```python
from build123d import *

# Parameters (mm, degrees)
SKETCH_1_R       = 8
EXTRUDE_1_DEPTH  = 24
SKETCH_2_R       = 17.5
SKETCH_2_R_2     = 8
EXTRUDE_2_DEPTH  = 18
EXTRUDE_3_DEPTH  = 18
EXTRUDE_4_DEPTH  = 18
EXTRUDE_5_DEPTH  = 18
EXTRUDE_6_DEPTH  = 18
EXTRUDE_7_DEPTH  = 18
EXTRUDE_8_DEPTH  = 18
EXTRUDE_9_DEPTH  = 18
EXTRUDE_10_DEPTH = 18
EXTRUDE_11_DEPTH = 18
EXTRUDE_12_DEPTH = 18
EXTRUDE_13_DEPTH = 18
EXTRUDE_14_DEPTH = 18
EXTRUDE_15_DEPTH = 18
EXTRUDE_16_DEPTH = 18
EXTRUDE_17_DEPTH = 18
EXTRUDE_18_DEPTH = 18
EXTRUDE_19_DEPTH = 18
EXTRUDE_20_DEPTH = 18
EXTRUDE_21_DEPTH = 18
EXTRUDE_22_DEPTH = 18


with BuildPart() as part:
    # 草图1 → 凸台-拉伸1 (new body)
    with BuildSketch(Plane.XY):
        Circle(SKETCH_1_R)
        with BuildLine():
            Line((4.520101179, 2.361924075), (-4.833937562, 1.62574526))
            ThreePointArc((-4.833937562, 1.62574526), (0.400141388, -5.084278402), (4.520101179, 2.361924075))
        make_face(mode=Mode.SUBTRACT)
    extrude(amount=EXTRUDE_1_DEPTH)

    # 草图2 → 凸台-拉伸2 (add)
    with BuildSketch(Plane.XY):
        Circle(SKETCH_2_R)
        Circle(SKETCH_2_R_2, mode=Mode.SUBTRACT)
    extrude(amount=EXTRUDE_2_DEPTH)

    # 草图3 → 凸台-拉伸3 (add)
    with BuildSketch(Plane.XY):
        with BuildLine():
            Line((17.423652167, 1.632894724), (21.989026862, 0.69476445))
            ThreePointArc((21.989026862, 0.69476445), (22, 0), (21.989026862, -0.69476445))
            Line((21.989026862, -0.69476445), (17.423652167, -1.632894724))
            ThreePointArc((17.423652167, -1.632894724), (17.5, 0), (17.423652167, 1.632894724))
        make_face()
    extrude(amount=EXTRUDE_3_DEPTH)

    # 草图4 → 凸台-拉伸4 (add)
    with BuildSketch(Plane.XY):
        with BuildLine():
            Line((16.066285711, 6.937179791), (20.698113262, 7.455743248))
            ThreePointArc((20.698113262, 7.455743248), (20.923243358, 6.798373876), (21.127501307, 6.134222733))
            Line((21.127501307, 6.134222733), (17.07547015, 3.831229456))
            ThreePointArc((17.07547015, 3.831229456), (16.643489035, 5.407797402), (16.066285711, 6.937179791))
        make_face()
    extrude(amount=EXTRUDE_4_DEPTH)

    # 草图5 → 凸台-拉伸5 (add)
    with BuildSketch(Plane.XY):
        with BuildLine():
            Line((13.13623927, 11.562405366), (17.381124124, 13.486901949))
            ThreePointArc((17.381124124, 13.486901949), (17.798373876, 12.93127555), (18.197868719, 12.362749455))
            Line((18.197868719, 12.362749455), (15.055822144, 8.920326203))
            ThreePointArc((15.055822144, 8.920326203), (14.157797402, 10.286241915), (13.13623927, 11.562405366))
        make_face()
    extrude(amount=EXTRUDE_5_DEPTH)

    # 草图6 → 凸台-拉伸6 (add)
    with BuildSketch(Plane.XY):
        with BuildLine():
            Line((8.920326203, 15.055822144), (12.212561116, 18.348057057))
            ThreePointArc((12.212561116, 18.348057057), (12.870731845, 17.892515435), (13.511927681, 17.413375811))
            Line((13.511927681, 17.413375811), (11.562405366, 13.13623927))
            ThreePointArc((11.562405366, 13.13623927), (10.286241915, 14.157797402), (8.920326203, 15.055822144))
        make_face()
    extrude(amount=EXTRUDE_6_DEPTH)

    # 草图7 → 凸台-拉伸7 (add)
    with BuildSketch(Plane.XY):
        with BuildLine():
            Line((3.831229456, 17.07547015), (6.134222733, 21.127501307))
            ThreePointArc((6.134222733, 21.127501307), (6.798373876, 20.923243358), (7.455743248, 20.698113262))
            Line((7.455743248, 20.698113262), (6.937179791, 16.066285711))
            ThreePointArc((6.937179791, 16.066285711), (5.407797402, 16.643489035), (3.831229456, 17.07547015))
        make_face()
    extrude(amount=EXTRUDE_7_DEPTH)

    # 草图8 → 凸台-拉伸8 (add)
    with BuildSketch(Plane.XY):
        with BuildLine():
            Line((-1.632894724, 17.423652167), (-0.69476445, 21.989026862))
            ThreePointArc((-0.69476445, 21.989026862), (0, 22), (0.69476445, 21.989026862))
            Line((0.69476445, 21.989026862), (1.632894724, 17.423652167))
            ThreePointArc((1.632894724, 17.423652167), (0, 17.5), (-1.632894724, 17.423652167))
        make_face()
    extrude(amount=EXTRUDE_8_DEPTH)

    # 草图9 → 凸台-拉伸9 (add)
    with BuildSketch(Plane.XY):
        with BuildLine():
            Line((-6.937179791, 16.066285711), (-7.455743248, 20.698113262))
            ThreePointArc((-7.455743248, 20.698113262), (-6.798373876, 20.923243358), (-6.134222733, 21.127501307))
            Line((-6.134222733, 21.127501307), (-3.831229456, 17.07547015))
            ThreePointArc((-3.831229456, 17.07547015), (-5.407797402, 16.643489035), (-6.937179791, 16.066285711))
        make_face()
    extrude(amount=EXTRUDE_9_DEPTH)

    # 草图10 → 凸台-拉伸10 (add)
    with BuildSketch(Plane.XY):
        with BuildLine():
            Line((-11.562405366, 13.13623927), (-13.486901949, 17.381124124))
            ThreePointArc((-13.486901949, 17.381124124), (-12.93127555, 17.798373876), (-12.362749455, 18.197868719))
            Line((-12.362749455, 18.197868719), (-8.920326203, 15.055822144))
            ThreePointArc((-8.920326203, 15.055822144), (-10.286241915, 14.157797402), (-11.562405366, 13.13623927))
        make_face()
    extrude(amount=EXTRUDE_10_DEPTH)

    # 草图11 → 凸台-拉伸11 (add)
    with BuildSketch(Plane.XY):
        with BuildLine():
            Line((-15.055822144, 8.920326203), (-18.348057057, 12.212561116))
            ThreePointArc((-18.348057057, 12.212561116), (-17.892515435, 12.870731845), (-17.413375811, 13.511927681))
            Line((-17.413375811, 13.511927681), (-13.13623927, 11.562405366))
            ThreePointArc((-13.13623927, 11.562405366), (-14.157797402, 10.286241915), (-15.055822144, 8.920326203))
        make_face()
    extrude(amount=EXTRUDE_11_DEPTH)

    # 草图12 → 凸台-拉伸12 (add)
    with BuildSketch(Plane.XY):
        with BuildLine():
            Line((-17.07547015, 3.831229456), (-21.127501307, 6.134222733))
            ThreePointArc((-21.127501307, 6.134222733), (-20.923243358, 6.798373876), (-20.698113262, 7.455743248))
            Line((-20.698113262, 7.455743248), (-16.066285711, 6.937179791))
            ThreePointArc((-16.066285711, 6.937179791), (-16.643489035, 5.407797402), (-17.07547015, 3.831229456))
        make_face()
    extrude(amount=EXTRUDE_12_DEPTH)

    # 草图13 → 凸台-拉伸13 (add)
    with BuildSketch(Plane.XY):
        with BuildLine():
            Line((-17.423652167, -1.632894724), (-21.989026862, -0.69476445))
            ThreePointArc((-21.989026862, -0.69476445), (-22, 0), (-21.989026862, 0.69476445))
            Line((-21.989026862, 0.69476445), (-17.423652167, 1.632894724))
            ThreePointArc((-17.423652167, 1.632894724), (-17.5, 0), (-17.423652167, -1.632894724))
        make_face()
    extrude(amount=EXTRUDE_13_DEPTH)

    # 草图14 → 凸台-拉伸14 (add)
    with BuildSketch(Plane.XY):
        with BuildLine():
            Line((-16.066285711, -6.937179791), (-20.698113262, -7.455743248))
            ThreePointArc((-20.698113262, -7.455743248), (-20.923243358, -6.798373876), (-21.127501307, -6.134222733))
            Line((-21.127501307, -6.134222733), (-17.07547015, -3.831229456))
            ThreePointArc((-17.07547015, -3.831229456), (-16.643489035, -5.407797402), (-16.066285711, -6.937179791))
        make_face()
    extrude(amount=EXTRUDE_14_DEPTH)

    # 草图15 → 凸台-拉伸15 (add)
    with BuildSketch(Plane.XY):
        with BuildLine():
            Line((-13.13623927, -11.562405366), (-17.381124124, -13.486901949))
            ThreePointArc((-17.381124124, -13.486901949), (-17.798373876, -12.93127555), (-18.197868719, -12.362749455))
            Line((-18.197868719, -12.362749455), (-15.055822144, -8.920326203))
            ThreePointArc((-15.055822144, -8.920326203), (-14.157797402, -10.286241915), (-13.13623927, -11.562405366))
        make_face()
    extrude(amount=EXTRUDE_15_DEPTH)

    # 草图16 → 凸台-拉伸16 (add)
    with BuildSketch(Plane.XY):
        with BuildLine():
            Line((-8.920326203, -15.055822144), (-12.212561116, -18.348057057))
            ThreePointArc((-12.212561116, -18.348057057), (-12.870731845, -17.892515435), (-13.511927681, -17.413375811))
            Line((-13.511927681, -17.413375811), (-11.562405366, -13.13623927))
            ThreePointArc((-11.562405366, -13.13623927), (-10.286241915, -14.157797402), (-8.920326203, -15.055822144))
        make_face()
    extrude(amount=EXTRUDE_16_DEPTH)

    # 草图17 → 凸台-拉伸17 (add)
    with BuildSketch(Plane.XY):
        with BuildLine():
            Line((-3.831229456, -17.07547015), (-6.134222733, -21.127501307))
            ThreePointArc((-6.134222733, -21.127501307), (-6.798373876, -20.923243358), (-7.455743248, -20.698113262))
            Line((-7.455743248, -20.698113262), (-6.937179791, -16.066285711))
            ThreePointArc((-6.937179791, -16.066285711), (-5.407797402, -16.643489035), (-3.831229456, -17.07547015))
        make_face()
    extrude(amount=EXTRUDE_17_DEPTH)

    # 草图18 → 凸台-拉伸18 (add)
    with BuildSketch(Plane.XY):
        with BuildLine():
            Line((1.632894724, -17.423652167), (0.69476445, -21.989026862))
            ThreePointArc((0.69476445, -21.989026862), (0, -22), (-0.69476445, -21.989026862))
            Line((-0.69476445, -21.989026862), (-1.632894724, -17.423652167))
            ThreePointArc((-1.632894724, -17.423652167), (0, -17.5), (1.632894724, -17.423652167))
        make_face()
    extrude(amount=EXTRUDE_18_DEPTH)

    # 草图19 → 凸台-拉伸19 (add)
    with BuildSketch(Plane.XY):
        with BuildLine():
            Line((6.937179791, -16.066285711), (7.455743248, -20.698113262))
            ThreePointArc((7.455743248, -20.698113262), (6.798373876, -20.923243358), (6.134222733, -21.127501307))
            Line((6.134222733, -21.127501307), (3.831229456, -17.07547015))
            ThreePointArc((3.831229456, -17.07547015), (5.407797402, -16.643489035), (6.937179791, -16.066285711))
        make_face()
    extrude(amount=EXTRUDE_19_DEPTH)

    # 草图20 → 凸台-拉伸20 (add)
    with BuildSketch(Plane.XY):
        with BuildLine():
            Line((11.562405366, -13.13623927), (13.486901949, -17.381124124))
            ThreePointArc((13.486901949, -17.381124124), (12.93127555, -17.798373876), (12.362749455, -18.197868719))
            Line((12.362749455, -18.197868719), (8.920326203, -15.055822144))
            ThreePointArc((8.920326203, -15.055822144), (10.286241915, -14.157797402), (11.562405366, -13.13623927))
        make_face()
    extrude(amount=EXTRUDE_20_DEPTH)

    # 草图21 → 凸台-拉伸21 (add)
    with BuildSketch(Plane.XY):
        with BuildLine():
            Line((15.055822144, -8.920326203), (18.348057057, -12.212561116))
            ThreePointArc((18.348057057, -12.212561116), (17.892515435, -12.870731845), (17.413375811, -13.511927681))
            Line((17.413375811, -13.511927681), (13.13623927, -11.562405366))
            ThreePointArc((13.13623927, -11.562405366), (14.157797402, -10.286241915), (15.055822144, -8.920326203))
        make_face()
    extrude(amount=EXTRUDE_21_DEPTH)

    # 草图22 → 凸台-拉伸22 (add)
    with BuildSketch(Plane.XY):
        with BuildLine():
            Line((17.07547015, -3.831229456), (21.127501307, -6.134222733))
            ThreePointArc((21.127501307, -6.134222733), (20.923243358, -6.798373876), (20.698113262, -7.455743248))
            Line((20.698113262, -7.455743248), (16.066285711, -6.937179791))
            ThreePointArc((16.066285711, -6.937179791), (16.643489035, -5.407797402), (17.07547015, -3.831229456))
        make_face()
    extrude(amount=EXTRUDE_22_DEPTH)


solid = part.part
```
Input: part model. Units: mm. Frame: model coordinates. A direction names the side the tool comes from. Round coordinates to 2 decimals unless told otherwise and drop trailing zeros. Write each loop counter-clockwise with the first axis right and the second up, starting at its lowest first coordinate (ties: lowest second). Pieces come first, ordered by that corner, then holes. Notation, with made-up numbers: (18, 70.25) -> (23, 70.25) arc R5 ccw to (23, 77.25) -> close; hole circle Ø5 at (38, -3). An arc over 180 degrees is marked (long way). Answer as CSV lines item,"result".
1. Reachability of faces 1 (the flat face through (4.967, 19.073, 8.874)), 2 (the cylindrical face through (-7.959, -15.586, 8.874)), 3 (the flat face through (5, -19.13, 8.87)), 4 (the flat face through (-9, 0, 18)) from +Z, -Z, +X, -X, +Y, -Y: full face, straight path, thin tool, end or side. Return the list, or none.
Geometry says:
face 1,"+Z, -Z, +Y"
face 2,"+Z, -Z"
face 3,"+Z, -Z, -Y"
face 4,"+Z"
2. Section C-C (y = -19). Return the cut outline in (x, z).
Geometry says:
outline,"(-7.27, 0) -> (-4.93, 0) -> (-4.93, 18) -> (-7.27, 18) -> close; (-1.31, 0) -> (1.31, 0) -> (1.31, 18) -> (-1.31, 18) -> close; (4.93, 0) -> (7.27, 0) -> (7.27, 18) -> (4.93, 18) -> close"
3. Ray query, L1, parallel to X at y = 0, z = 5.25; L2, parallel to X at y = -12.5, z = 8; L3, parallel to Z at x = -15, y = 8.5. Return the intervals inside material, ascending. Write a range as [from, to].
Geometry says:
L1,"x = [-22, -5.1], [5.1, 22]"
L2,"x = [-18.1, -15.2], [-12.25, 12.25], [15.19, 18.15]"
L3,"z = [0, 18]"
4. Section D-D (z = 19.75). Return the cut outline in (x, y), plus the area to 3 significant figures.
Geometry says:
outline,"circle Ø16 at (0, 0); hole (-4.83, 1.63) arc R5.1 ccw (long way) to (4.52, 2.36) -> close"
area,"140 mm^2"
5. Section B-B (x = 0). Return the cut outline in (y, z), plus the area to 3 significant figures.
Geometry says:
outline,"(-22, 0) -> (-5.1, 0) -> (-5.1, 24) -> (-8, 24) -> (-8, 18) -> (-22, 18) -> close; (2.01, 0) -> (22, 0) -> (22, 18) -> (8, 18) -> (8, 24) -> (2.01, 24) -> close"
area,"717 mm^2"
6. Mould query, pull axis X, two halves, no side actions, for faces 5 (the cylindrical face through (12.86, 17.9, 8.87)), 6 (the cylindrical face through (-17.9, 12.86, 8.87)), 7 (the flat face through (1.157, 19.738, 8.874)). Classes: +X half, -X half, draft (parallel to the pull), parting line (faces both ways), or undercut.
Geometry says:
face 5,"+X half"
face 6,"-X half"
face 7,"undercut"
7. Contact query for flat-ended pins moving along their axis: P1, Ø2, axis at y = 13.5, z = 16.5, coming from the +X side; P2, Ø8, axis at x = 8, y = -16, coming from the +Z side; P3, Ø6, axis at x = 7, z = 11.5, coming from the -Y side. Output: stop coordinate, or through.
Geometry says:
P1,"stops at x = 18.1"
P2,"stops at z = 18"
P3,"stops at y = -21.13"
8. Section A-A (y = 0). Return the cut outline in (x, z), plus the area to 3 significant figures.
Geometry says:
outline,"(-22, 0) -> (-5.1, 0) -> (-5.1, 24) -> (-8, 24) -> (-8, 18) -> (-22, 18) -> close; (5.1, 0) -> (22, 0) -> (22, 18) -> (8, 18) -> (8, 24) -> (5.1, 24) -> close"
area,"643 mm^2"
